```python
from build123d import *

# Parameters (mm, degrees)
F0_W     = 50
F0_H     = 20
F0_R     = 4
F0_W_2   = 20
F0_W_3   = 140
F1_DEPTH = 15
F0_H_2   = 10
F2_DEPTH = 30
F3_SIZE  = 9.99999


# Not quite as in the source:
# - a fillet or chamfer is up to 0.001 mm smaller than in the source, because OpenCascade refuses the exact size
# - a feature names something its author has since deleted; it is built from what else it names


with BuildPart() as f1:
    # F0 (on Front) → F1 (new body)
    with BuildSketch(Plane.XZ):
        with Locations((-115, 10)):
            Rectangle(F0_W, F0_H)
        with Locations((-96.25, 10)):
            Circle(F0_R, mode=Mode.SUBTRACT)
        with Locations((-80, 10)):
            Rectangle(F0_W_2, F0_H)
        with Locations((80, 10)):
            Rectangle(F0_W_2, F0_H)
        with Locations((115, 10)):
            Rectangle(F0_W, F0_H)
        with Locations((96.25, 10)):
            Circle(F0_R, mode=Mode.SUBTRACT)
        with Locations((0, 10)):
            Rectangle(F0_W_3, F0_H)
        with Locations((-63.75, 10)):
            Circle(F0_R, mode=Mode.SUBTRACT)
        with Locations((-16.25, 10)):
            Circle(F0_R, mode=Mode.SUBTRACT)
        with Locations((16.25, 10)):
            Circle(F0_R, mode=Mode.SUBTRACT)
        with Locations((63.75, 10)):
            Circle(F0_R, mode=Mode.SUBTRACT)
    extrude(amount=F1_DEPTH)

    # F0 (on Front) → F2 (join)
    with BuildSketch(Plane.XZ):
        with Locations((80, 25)):
            Rectangle(F0_W_2, F0_H_2)
        with Locations((-80, 25)):
            Rectangle(F0_W_2, F0_H_2)
        with Locations((-80, -5)):
            Rectangle(F0_W_2, F0_H_2)
        with Locations((80, -5)):
            Rectangle(F0_W_2, F0_H_2)
    extrude(amount=F2_DEPTH)

    # F3 (size 10 in the source; OpenCascade refuses exactly that, so slightly less here)
    f3_edges = [f1.edges().sort_by_distance(p)[0] for p in [
        (70, -7.5, 20),
        (90, -7.5, 20),
        (-70, -7.5, 20),
        (-90, -7.5, 20),
        (-90, -7.5, 0),
        (-70, -7.5, 0),
        (70, -7.5, 0),
        (90, -7.5, 0),
    ]]
    chamfer(f3_edges, length=F3_SIZE)


solid = f1.part
```
Model file for the job. Use its own axes, mm. A direction names the side the tool comes from. Coordinates: 2 decimals unless noted, no trailing zeros. Write each loop counter-clockwise with the first axis right and the second up, starting at its lowest first coordinate (ties: lowest second). Pieces come first, ordered by that corner, then holes. Notation, with made-up numbers: (20.5, 43) - (36.5, 43) arc R21 ccw to (36.5, 56) - close; hole circle Ø8 at (-12, -16). An arc over 180 degrees is marked (long way). One line per question, with ' | ' between items. Start each with the question number.
Q1. 3-axis set-ups, long thin cutter, end or side, ignore diameter. For faces 4 (the face through (90, -25, -5)), 5 (the face through (120, -7, 0)), 6 (the face through (-80, -22, 0)), 7 (the face through (-20.246, -7.395, 10.176)): which of +Z, -Z, +X, -X, +Y, -Y reach the whole face in a straight line?
Q2. Cut at A-A, the plane y = -22.75. List the corners of the cut face in (x, z), then the cut area to 3 significant figures.
Q3. Cut at C-C, the plane z = 10. List the corners of the cut face in (x, y).
Q4. Drill centre lines: line 1 (Z direction, x = -16.25, y = -5.5); line 2 (Z direction, x = 87, y = -15.75); line 3 (X direction, y = -19.75, z = -3). Where is each one in solid material? Low to high. Write a range as [from, to].
Q5. Pull direction Z, two halves, no side cores. Call faces 1 (the face through (120, -7, 20)), 2 (the face through (-90, -25, -5)), 3 (the face through (80, -22, 0)): pulls with the +Z half, pulls with the -Z half, needs draft (parallel to the pull), parting line crosses it, or undercut.
Q6. Cut at D-D, the plane z = 24.5. List the corners of the cut face in (x, y), then the cut area to 3 significant figures.
Q7. Cut at B-B, the plane x = 16.25. List the corners of the cut face in (y, z), then the cut area to 3 significant figures.
Q8. Pin check, flat tips, straight feed: pin 1 (12 mm diameter, centred on x = -44, z = 22.5, fed in from +Y); pin 2 (4 mm diameter, centred on y = -21, z = 18.5, fed in from +X); pin 3 (12 mm diameter, centred on x = 121.5, y = -8, fed in from -Z); pin 4 (2 mm diameter, centred on y = -4.5, z = 22, fed in from -X). Stop position of each tip, or through.
Answer below:
1) face 4: +Z, -Z, +X, -Y | face 5: -Z, +X, +Y, -Y | face 6: +X, -X, -Y | face 7: +Y, -Y
2) outline: (-90, -10) - (-70, -10) - (-70, 0) - (-90, 0) - close; (-90, 20) - (-70, 20) - (-70, 30) - (-90, 30) - close; (70, -10) - (90, -10) - (90, 0) - (70, 0) - close; (70, 20) - (90, 20) - (90, 30) - (70, 30) - close | area: 800 mm^2
3) outline: (-140, -15) - (-100.25, -15) - (-100.25, 0) - (-140, 0) - close; (-92.25, -15) - (-67.75, -15) - (-67.75, 0) - (-92.25, 0) - close; (-59.75, -15) - (-20.25, -15) - (-20.25, 0) - (-59.75, 0) - close; (-12.25, -15) - (12.25, -15) - (12.25, 0) - (-12.25, 0) - close; (20.25, -15) - (59.75, -15) - (59.75, 0) - (20.25, 0) - close; (67.75, -15) - (92.25, -15) - (92.25, 0) - (67.75, 0) - close; (100.25, -15) - (140, -15) - (140, 0) - (100.25, 0) - close
4) line 1: [0, 6], [14, 20] | line 2: [-10, 0], [20, 30] | line 3: [-90, -70], [70, 90]
5) face 1: pulls with the +Z half | face 2: needs draft | face 3: undercut
6) outline: (-95.5, -15) - (-90, -15) - (-90, -30) - (-70, -30) - (-70, -15) - (-64.5, -15) - (-64.5, 0) - (-95.5, 0) - close; (64.5, -15) - (70, -15) - (70, -30) - (90, -30) - (90, -15) - (95.5, -15) - (95.5, 0) - (64.5, 0) - close | area: 1,530 mm^2
7) outline: (-15, 0) - (0, 0) - (0, 6) - (-15, 6) - close; (-15, 14) - (0, 14) - (0, 20) - (-15, 20) - close | area: 180 mm^2
8) pin 1: y = 0 | pin 2: x = 90 | pin 3: z = 0 | pin 4: x = -99
